Design review of the part built by this model. Coordinates are the model's own, in mm. A direction names the side the tool comes from. Round coordinates to 2 decimals unless told otherwise and drop trailing zeros. Loops run counter-clockwise (first coordinate to the right, second up) from the corner with the lowest first, then second, coordinate; pieces in that order, holes last. Notation, with made-up numbers: (28.25, 37) - (68.25, 37) arc R23 ccw to (68.25, 59) - close; hole circle Ø3 at (48, 57.5). An arc over 180 degrees is marked (long way). Return JSON: item names as keys, results as strings. Group by question number.
(1) Wall thickness on L1, parallel to Z at x = 42, y = 41; L2, parallel to Y at x = 49, z = -1.5: over which ranges is each line inside the solid? List them lowest first. Write a range as [from, to].
(2) We need section A-A, the plane y = 34. Write out the cut boundary in (x, z), and give its area (3 significant figures).
(3) Clearance check with a flat-ended pin moving along its axis: pin 1 (12 mm diameter, centred on x = 3.5, z = -12, fed in from +Y). State where the tip first meets the part, or that it passes through.
(4) We need section B-B, the plane x = 66.5. Write out the cut boundary in (y, z), and give its area (3 significant figures).
(5) For faces 5 (the flat face through (-1, 31, -44.759)), 6 (the flat face through (-1, 0, -1)), list the 3-axis set-ups (+Z, -Z, +X, -X, +Y, -Y) from which the entire face can be reached by the end or side of a thin tool; tool diameter is ignored.
(6) We need section C-C, the plane z = 21.5. Write out the cut boundary in (x, y), and give its area (3 significant figures).
(7) The part is to be moulded in two halves that separate along Z. For faces 1 (the flat face through (-1, 26, 54.759)), 2 (the flat face through (-1, 26, -54.759)), 3 (the flat face through (-1, 51.086, 50)), 4 (the flat face through (-1, 31, 44.759)), say which applies: pulls with the +Z half, pulls with the -Z half, needs draft (parallel to the pull), parting line crosses it, or undercut.
from build123d import *

# Parameters (mm, degrees)
SKETCH1_W           = 162.841056138
SKETCH1_H           = 109.517788384
BOSS_EXTRUDE1_DEPTH = 10
SKETCH3_W           = 162.841056138
SKETCH3_H           = 41.085879715
BOSS_EXTRUDE2_DEPTH = 10


with BuildPart() as part:
    # Sketch1 → Boss-Extrude1 (new body)
    with BuildSketch(Plane(origin=(0, 0, 0), x_dir=(1, 0, 0), z_dir=(0, 1, 0))):
        Rectangle(SKETCH1_W, SKETCH1_H)
    extrude(amount=BOSS_EXTRUDE1_DEPTH)

    # Sketch3 → Boss-Extrude2 (add)
    with BuildSketch(Plane.XY.offset(54.758894192)):
        with Locations((0, 30.542939858)):
            Rectangle(SKETCH3_W, SKETCH3_H)
    boss_extrude2 = extrude(amount=-BOSS_EXTRUDE2_DEPTH)

    # Mirror1: Boss-Extrude2 across plane
    add(boss_extrude2.mirror(Plane.XY))


solid = part.part
Solutions:
{
 "1": {"L1": "[-54.76, -44.76], [44.76, 54.76]", "L2": "[0, 10]"},
 "2": {"outline": "(-81.42, -54.76) - (81.42, -54.76) - (81.42, -44.76) - (-81.42, -44.76) - close; (-81.42, 44.76) - (81.42, 44.76) - (81.42, 54.76) - (-81.42, 54.76) - close", "area": "3,260 mm^2"},
 "3": {"pin 1": "y = 10"},
 "4": {"outline": "(0, -54.76) - (51.09, -54.76) - (51.09, -44.76) - (10, -44.76) - (10, 44.76) - (51.09, 44.76) - (51.09, 54.76) - (0, 54.76) - close", "area": "1,920 mm^2"},
 "5": {"face 5": "+X, -X, +Y", "face 6": "+Z, -Z, +X, -X, -Y"},
 "6": {"outline": "(-81.42, 0) - (81.42, 0) - (81.42, 10) - (-81.42, 10) - close", "area": "1,630 mm^2"},
 "7": {"face 1": "pulls with the +Z half", "face 2": "pulls with the -Z half", "face 3": "needs draft", "face 4": "undercut"}
}
